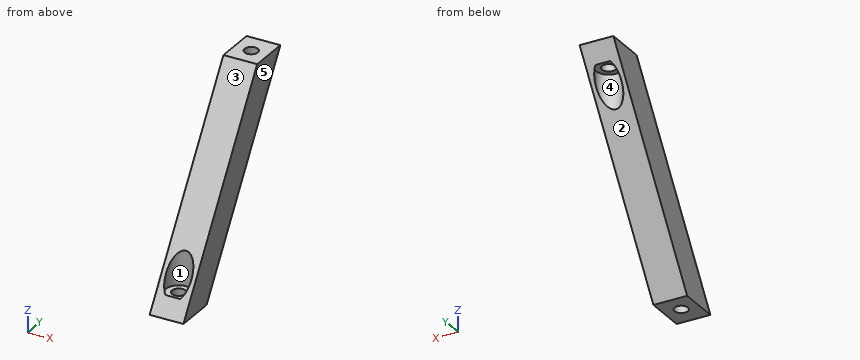
```python
from build123d import *

# Parameters (mm, degrees)
BOSS_EXTRUDE1_DEPTH = 20
SKETCH2_R           = 4
CUT_EXTRUDE5_DEPTH  = 117
CUT_EXTRUDE6_START  = -10
SKETCH5_R           = 7.5
CUT_EXTRUDE6_DEPTH  = 107
SKETCH6_R           = 4
CUT_EXTRUDE7_DEPTH  = 117
CUT_EXTRUDE8_START  = -10
SKETCH7_R           = 7.5
CUT_EXTRUDE8_DEPTH  = 107


with BuildPart() as part:
    # Sketch1 → Boss-Extrude1 (new body)
    with BuildSketch(Plane(origin=(0, 0, 0), x_dir=(0, 0, -1), z_dir=(1, 0, 0))):
        Polygon((116, 48.213061677), (0, 124.295055109), (0, 100.377048541), (116, 24.295055109), align=None)
    extrude(amount=BOSS_EXTRUDE1_DEPTH)

    # Sketch2 → Cut-Extrude5 (cut, through all)
    with BuildSketch(Plane.XY):
        with Locations((10, 111.680172571)):
            Circle(SKETCH2_R)
    extrude(amount=-CUT_EXTRUDE5_DEPTH, mode=Mode.SUBTRACT)

    # Sketch5 → Cut-Extrude6 (cut, through all)
    with BuildSketch(Plane.XY.offset(CUT_EXTRUDE6_START)):
        with Locations((10, 111.680172571)):
            Circle(SKETCH5_R)
    extrude(amount=-CUT_EXTRUDE6_DEPTH, mode=Mode.SUBTRACT)

    # Sketch6 → Cut-Extrude7 (cut, through all)
    with BuildSketch(Plane(origin=(0, 0, -116), x_dir=(-1, 0, 0), z_dir=(0, 0, -1))):
        with Locations((-10, 36.909937646)):
            Circle(SKETCH6_R)
    extrude(amount=-CUT_EXTRUDE7_DEPTH, mode=Mode.SUBTRACT)

    # Sketch7 → Cut-Extrude8 (cut, through all)
    with BuildSketch(Plane(origin=(0, 0, -116), x_dir=(-1, 0, 0), z_dir=(0, 0, -1)).offset(CUT_EXTRUDE8_START)):
        with Locations((-10, 36.909937646)):
            Circle(SKETCH7_R)
    extrude(amount=-CUT_EXTRUDE8_DEPTH, mode=Mode.SUBTRACT)


solid = part.part
```
Design review of the part built by this model. Coordinates are the model's own, in mm. Face numbers are marked on the shaded views. A direction names the side the tool comes from. Coordinates: 2 decimals unless noted, no trailing zeros. Order: outer loops, then holes, each group sorted by start corner. A loop starts at its lowest first (then second) coordinate and runs counter-clockwise, first axis right, second up. Notation, with made-up numbers: M -25,21.5 L 16,21.5 A29 cw 16,58.5 Z; hole C 66.25,2 d10. An arc over 180 degrees is marked long. Answer as a JSON object with one key per item and string values. Group by question number.
1) Mouldability with a two-part tool opening along Y and no side actions: class the marked faces 1, 2 and 3 as pulls with the +Y half, pulls with the -Y half, needs draft (parallel to the pull), parting line crosses it, or undercut.
2) Add section D-D, the plane y = 102. Write out the cut boundary in (x, z), then the cut area to 3 significant figures.
3) For pin 1 (2 mm diameter, centred on x = 5, y = 94.5, fed in from -Z); pin 2 (2 mm diameter, centred on x = 4.5, y = 56, fed in from -Z); pin 3 (12 mm diameter, centred on x = 10, y = 43, fed in from +Z); pin 4 (10.5 mm diameter, centred on x = 10, y = 111.68, fed in from +Z), all flat-tipped, find the tip position at first contact; note any pin that passes through.
4) Add section C-C, the plane z = -14.5. Write out the cut boundary in (x, y), then the cut area to 3 significant figures.
5) Wall thickness on L1, parallel to Z at x = 3.25, y = 38.5; L2, parallel to X at y = 40, z = -102.5; L3, parallel to X at y = 107.5, z = -14.5: over which ranges is each line inside the solid? List them lowest first.
6) Tool access review of the marked faces 4 and 5: name each direction out of +Z, -Z, +X, -X, +Y, -Y from which nothing blocks a thin tool from reaching the whole face with its end or side.
7) Add section B-B, the plane y = 113. Write out the cut boundary in (x, z), then the cut area to 3 significant figures.
8) Add section A-A, the plane x = 10. Write out the cut boundary in (y, z).
Computed values:
{
 "1": {"face 1": "undercut", "face 2": "pulls with the +Y half", "face 3": "pulls with the -Y half"},
 "2": {"outline": "M 0,-33.99 L 20,-33.99 L 20,0 L 0,0 Z", "area": "680 mm^2"},
 "3": {"pin 1": "stops at z = -46.95", "pin 2": "stops at z = -105.65", "pin 3": "stops at z = -78.33", "pin 4": "stops at z = 0"},
 "4": {"outline": "M 0,90.87 L 20,90.87 L 20,114.78 L 16.83,114.78 A7.5 cw long 3.17,114.78 L 0,114.78 Z", "area": "345 mm^2"},
 "5": {"L1": "z = -116 to -106", "L2": "x = 0 to 3.17, 16.83 to 20", "L3": "x = 0 to 3.77, 16.23 to 20"},
 "6": {"face 4": "-Z", "face 5": "+Z, -Z, +X, +Y, -Y"},
 "7": {"outline": "M 0,-17.22 L 2.62,-17.22 L 2.62,-10 L 6.22,-10 L 6.22,0 L 0,0 Z; M 13.78,-10 L 17.38,-10 L 17.38,-17.22 L 20,-17.22 L 20,0 L 13.78,0 Z", "area": "162 mm^2"},
 "8": {"outline": "M 24.3,-116 L 32.91,-116 L 32.91,-106 L 30.85,-106 Z; M 40.91,-116 L 48.21,-116 L 104.18,-30.67 L 104.18,-10 L 107.68,-10 L 107.68,0 L 100.38,0 L 44.41,-85.33 L 44.41,-106 L 40.91,-106 Z; M 115.68,-10 L 117.74,-10 L 124.3,0 L 115.68,0 Z"}
}
